For this review, take the finished solid that the model builds, in its own axes (mm). Give positions to 0.01 mm unless a question says otherwise; leave off trailing zeros. Loops run counter-clockwise (first coordinate to the right, second up) from the corner with the lowest first, then second, coordinate; pieces in that order, holes last. Notation, with made-up numbers: (20.25, 54.5) - (42.25, 54.5) arc R20 cw to (42.25, 80.5) - close; hole circle Ø1 at (73.25, 5). An arc over 180 degrees is marked (long way). Answer in a Markdown table with one row per item.
```python
from build123d import *

# Parameters (mm, degrees)
F0_W     = 25
F0_H     = 25
F1_DEPTH = 3.175
F0_W_2   = 173.35
F0_H_2   = 143.35
F2_DEPTH = 9.525
F3_W     = 137
F3_H     = 3.175
F4_DEPTH = 25.4
F5_W     = 167
F5_H     = 3.175
F6_DEPTH = 1.5875
F7_W     = 167
F7_H     = 3.175
F8_DEPTH = 1.5875


with BuildPart() as f1:
    # F0 (on Top) → F1 (new body)
    with BuildSketch(Plane.XY):
        Polygon((-41.7, 68.5), (-67.1, 68.5), (-83.5, 68.5), (-83.5, 52.1), (-83.5, 26.7), (-83.5, -24.1), (-83.5, -49.5), (-83.5, -68.5), (-67.1, -68.5), (-41.7, -68.5), (-16.3, -68.5), (9.1, -68.5), (34.5, -68.5), (59.9, -68.5), (83.5, -68.5), (83.5, -49.5), (83.5, -24.1), (83.5, 26.7), (83.5, 52.1), (83.5, 68.5), (59.9, 68.5), (34.5, 68.5), (9.1, 68.5), (-16.3, 68.5), align=None)
        Rectangle(F0_W, F0_H, mode=Mode.SUBTRACT)
    extrude(amount=F1_DEPTH)

    # F0 (on Top) → F2 (join)
    with BuildSketch(Plane.XY):
        Rectangle(F0_W_2, F0_H_2)
        Polygon((-83.5, 68.5), (-67.1, 68.5), (-41.7, 68.5), (-16.3, 68.5), (9.1, 68.5), (34.5, 68.5), (59.9, 68.5), (83.5, 68.5), (83.5, 52.1), (83.5, 26.7), (83.5, -24.1), (83.5, -49.5), (83.5, -68.5), (59.9, -68.5), (34.5, -68.5), (9.1, -68.5), (-16.3, -68.5), (-41.7, -68.5), (-67.1, -68.5), (-83.5, -68.5), (-83.5, -49.5), (-83.5, -24.1), (-83.5, 26.7), (-83.5, 52.1), align=None, mode=Mode.SUBTRACT)
    extrude(amount=F2_DEPTH)

    # F3 (on face) → F4 (cut)
    with BuildSketch(Plane.YZ.offset(-83.5)):
        with Locations((0, 4.7625)):
            Rectangle(F3_W, F3_H)
    extrude(amount=-F4_DEPTH, mode=Mode.SUBTRACT)

    # F5 (on face) → F6 (join)
    with BuildSketch(Plane.XZ.offset(-68.5)):
        with Locations((0, 7.9375)):
            Rectangle(F5_W, F5_H)
    extrude(amount=F6_DEPTH)

    # F7 (on face) → F8 (join)
    with BuildSketch(Plane(origin=(0, -68.5, 0), x_dir=(-1, 0, 0), z_dir=(0, 1, 0))):
        with Locations((0, 7.9375)):
            Rectangle(F7_W, F7_H)
    extrude(amount=F8_DEPTH)


solid = f1.part
```
1. Clearance check with a flat-ended pin moving along its axis: pin 1 (3 mm diameter, centred on x = 69, y = 11.5, fed in from +Z) (3 decimals). State where the tip first meets the part, or that it passes through.
Values:
| item | result |
|---|---|
| pin 1 | stops at z = 3.175 |
2. Wall thickness on line 1 (Y direction, x = 28, z = 5) (3 decimals); line 2 (Y direction, x = 63, z = 7.25) (1 decimal); line 3 (X direction, y = 13.5, z = 6.75) (3 decimals): over which ranges is each line inside the solid? List them lowest first. Write a range as [from, to].
Values:
| item | result |
|---|---|
| line 1 | y = [-71.675, -68.5], [68.5, 71.675] |
| line 2 | y = [-71.7, -66.9], [66.9, 71.7] |
| line 3 | x = [-86.675, -83.5], [83.5, 86.675] |
3. We need section A-A, the plane y = 5. Give the boundary of the cut face in (x, z) (3 decimals).
Values:
| item | result |
|---|---|
| outline | (-86.675, 0) - (-12.5, 0) - (-12.5, 3.175) - (-86.675, 3.175) - close; (-86.675, 6.35) - (-83.5, 6.35) - (-83.5, 9.525) - (-86.675, 9.525) - close; (12.5, 0) - (86.675, 0) - (86.675, 9.525) - (83.5, 9.525) - (83.5, 3.175) - (12.5, 3.175) - close |
4. Mouldability with a two-part tool opening along X and no side actions: class faces 1 (the face through (-1, 71.675, 5)), 2 (the face through (-86.675, -1, 3)), 3 (the face through (83.5, 1, 6)), 4 (the face through (86.675, -1, 5)) as released by +X, released by -X, zero draft, split by the parting line, or undercut.
Values:
| item | result |
|---|---|
| face 1 | zero draft |
| face 2 | released by -X |
| face 3 | undercut |
| face 4 | released by +X |
5. We need section C-C, the plane y = 57.5. Give the boundary of the cut face in (x, z) (3 decimals).
Values:
| item | result |
|---|---|
| outline | (-86.675, 0) - (86.675, 0) - (86.675, 9.525) - (83.5, 9.525) - (83.5, 3.175) - (-86.675, 3.175) - close; (-86.675, 6.35) - (-83.5, 6.35) - (-83.5, 9.525) - (-86.675, 9.525) - close |
